Geometry check sheet. Reference: drawing and pictorial views, mm from the part's lowest x, y, z. A direction names the side the tool comes from. Coordinates: 2 decimals unless noted, no trailing zeros. Write each loop counter-clockwise with the first axis right and the second up, starting at its lowest first coordinate (ties: lowest second). Pieces come first, ordered by that corner, then holes.
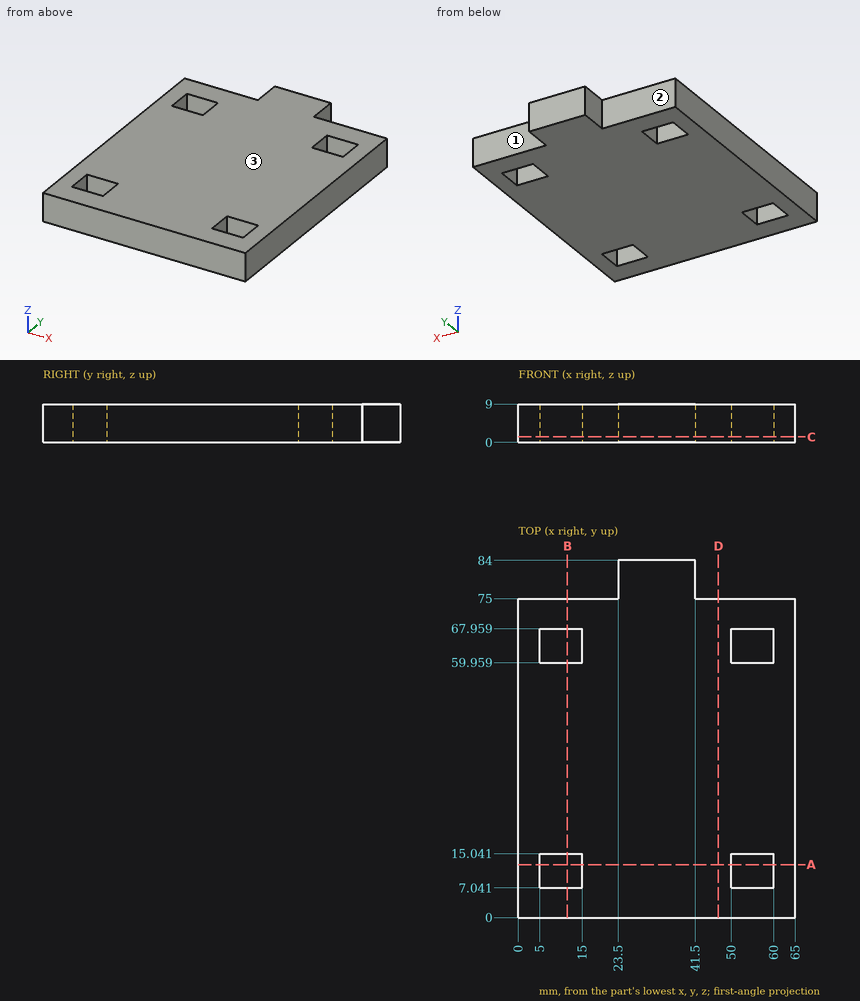
1. Sectioned sample at B-B, the plane x = 11.5. Record the boundary of the cut face in (y, z), and give its area (3 significant figures).
2. Tool access check on the marked faces 1, 2 and 3. Record the directions out of +Z, -Z, +X, -X, +Y, -Y that give a thin tool (end or side, any length) a straight path to the whole face; none if there is none.
3. Sectioned sample at D-D, the plane x = 47. Record the boundary of the cut face in (y, z), and give its area (3 significant figures).
4. Material ranges on L1, parallel to Y at x = 7.5, z = 6.25; L2, parallel to X at y = 9.5, z = 8; L3, parallel to Y at x = 49, z = 1, recorded low to high.
5. Sectioned sample at A-A, the plane y = 12.5. Record the boundary of the cut face in (x, z), and give its area (3 significant figures).
6. Gauge pin test, flat ends, axial feed: P1, Ø2.5, axis at x = 55, z = 4, coming from the +Y side; P2, Ø2.5, axis at y = 78, z = 6, coming from the -X side. Record the tip position at first contact, or that the pin passes through.
7. Sectioned sample at C-C, the plane z = 1.25. Record the boundary of the cut face in (x, y).
Outcome:
1. outline: (0, 0) - (7.04, 0) - (7.04, 9) - (0, 9) - close; (15.04, 0) - (59.96, 0) - (59.96, 9) - (15.04, 9) - close; (67.96, 0) - (75, 0) - (75, 9) - (67.96, 9) - close
1. area: 531 mm2
2. face 1: +Z, -Z, +X, +Y
2. face 2: +Z, -Z, -X, +Y
2. face 3: +Z, +X, -X, +Y, -Y
3. outline: (0, 0) - (75, 0) - (75, 9) - (0, 9) - close
3. area: 675 mm2
4. L1: y = 0 to 7.04, 15.04 to 59.96, 67.96 to 75
4. L2: x = 0 to 5, 15 to 50, 60 to 65
4. L3: y = 0 to 75
5. outline: (0, 0) - (5, 0) - (5, 9) - (0, 9) - close; (15, 0) - (50, 0) - (50, 9) - (15, 9) - close; (60, 0) - (65, 0) - (65, 9) - (60, 9) - close
5. area: 405 mm2
6. P1: stops at y = 75
6. P2: stops at x = 23.5
7. outline: (0, 0) - (65, 0) - (65, 75) - (41.5, 75) - (41.5, 84) - (23.5, 84) - (23.5, 75) - (0, 75) - close; hole (5, 7.04) - (15, 7.04) - (15, 15.04) - (5, 15.04) - close; hole (5, 59.96) - (15, 59.96) - (15, 67.96) - (5, 67.96) - close; hole (50, 7.04) - (60, 7.04) - (60, 15.04) - (50, 15.04) - close; hole (50, 59.96) - (60, 59.96) - (60, 67.96) - (50, 67.96) - close
